The listing builds one solid part. Answer for the finished solid, in the listing's coordinates (mm). A direction names the side the tool comes from. Coordinates: 2 decimals unless noted, no trailing zeros. Order: outer loops, then holes, each group sorted by start corner. A loop starts at its lowest first (then second) coordinate and runs counter-clockwise, first axis right, second up. Notation, with made-up numbers: (69.5, 53.5) -> (104.5, 53.5) arc R19 cw to (104.5, 58.5) -> close; hole circle Ø2 at (6, -33). An arc over 180 degrees is marked (long way). Put each result on its own line as item: value. Start each with the question number.
```python
from build123d import *

# Parameters (mm, degrees)
EXTRUDE_1_DEPTH     = 1.63
SKETCH_2_R          = 1.5
CUT_EXTRUDE_1_DEPTH = 1.6
SKETCH_3_W          = 29.19
SKETCH_3_H          = 26.15
EXTRUDE_2_DEPTH     = 1.8
EXTRUDE_3_DEPTH     = 2
SKETCH_6_W          = 3
SKETCH_6_H          = 26.15
CUT_EXTRUDE_2_DEPTH = 0.2
SKETCH_4_W          = 5.81
SKETCH_4_H          = 3.67
EXTRUDE_4_DEPTH     = 2
SKETCH_7_W          = 2.6
SKETCH_7_H          = 1.3
EXTRUDE_5_DEPTH     = 1
SKETCH_8_W          = 51
SKETCH_8_H          = 5
EXTRUDE_6_DEPTH     = 3.68
SKETCH_9_W          = 1.9
SKETCH_9_H          = 1.9
EXTRUDE_7_DEPTH     = 3
SKETCH_10_R         = 1.6
EXTRUDE_8_DEPTH     = 1


with BuildPart() as part:
    # 草图1 → 凸台-拉伸1 (new body)
    with BuildSketch(Plane(origin=(0, 0, 0), x_dir=(1, 0, 0), z_dir=(0, 1, 0))):
        with BuildLine():
            Line((-29.5, 15.375), (29.5, 15.375))
            ThreePointArc((29.5, 15.375), (31.621320344, 14.496320344), (32.5, 12.375))
            Line((32.5, 12.375), (32.5, -12.375))
            ThreePointArc((32.5, -12.375), (31.621320344, -14.496320344), (29.5, -15.375))
            Line((29.5, -15.375), (-29.5, -15.375))
            ThreePointArc((-29.5, -15.375), (-31.621320344, -14.496320344), (-32.5, -12.375))
            Line((-32.5, -12.375), (-32.5, 12.375))
            ThreePointArc((-32.5, 12.375), (-31.621320344, 14.496320344), (-29.5, 15.375))
        make_face()
    extrude(amount=EXTRUDE_1_DEPTH)

    # 草图2 → 切除-拉伸1 (cut)
    with BuildSketch(Plane(origin=(0, 1.63, 0), x_dir=(1, 0, 0), z_dir=(0, 1, 0))):
        with Locations(Location((-29, 11.875, 0), (0, 0, 270))):
            Circle(SKETCH_2_R)
        with Locations(Location((-29, -11.875, 0), (0, 0, 270))):
            Circle(SKETCH_2_R)
        with Locations(Location((29, -11.875, 0), (0, 0, 270))):
            Circle(SKETCH_2_R)
        with Locations(Location((29, 11.875, 0), (0, 0, 270))):
            Circle(SKETCH_2_R)
    extrude(amount=-CUT_EXTRUDE_1_DEPTH, mode=Mode.SUBTRACT)

    # 草图3 → 凸台-拉伸2 (add)
    with BuildSketch(Plane(origin=(0, 1.63, 0), x_dir=(1, 0, 0), z_dir=(0, 1, 0))):
        with Locations((0.765, 1.1)):
            Rectangle(SKETCH_3_W, SKETCH_3_H)
    extrude(amount=EXTRUDE_2_DEPTH)

    # 草图5 → 凸台-拉伸3 (add)
    with BuildSketch(Plane(origin=(0, 1.63, 0), x_dir=(1, 0, 0), z_dir=(0, 1, 0))):
        with BuildLine():
            Line((26.574695167, 4.138250353), (29.014213562, 1.698731957))
            ThreePointArc((29.014213562, 1.698731957), (29.6, 0.284518395), (29.014213562, -1.129695167))
            Line((29.014213562, -1.129695167), (26.574695167, -3.569213562))
            ThreePointArc((26.574695167, -3.569213562), (25.160481605, -4.155), (23.746268043, -3.569213562))
            Line((23.746268043, -3.569213562), (21.306749647, -1.129695167))
            ThreePointArc((21.306749647, -1.129695167), (20.72096321, 0.284518395), (21.306749647, 1.698731957))
            Line((21.306749647, 1.698731957), (23.746268043, 4.138250353))
            ThreePointArc((23.746268043, 4.138250353), (25.160481605, 4.72403679), (26.574695167, 4.138250353))
        make_face()
    extrude(amount=EXTRUDE_3_DEPTH)

    # 草图6 → 切除-拉伸2 (cut)
    with BuildSketch(Plane(origin=(0, 3.43, 0), x_dir=(1, 0, 0), z_dir=(0, 1, 0))):
        with Locations((-12.33, 1.1)):
            Rectangle(SKETCH_6_W, SKETCH_6_H)
    extrude(amount=-CUT_EXTRUDE_2_DEPTH, mode=Mode.SUBTRACT)

    # 草图4 → 凸台-拉伸4 (add)
    with BuildSketch(Plane(origin=(0, 1.63, 0), x_dir=(1, 0, 0), z_dir=(0, 1, 0))):
        with Locations((-24.325, 6.14)):
            Rectangle(SKETCH_4_W, SKETCH_4_H)
        with Locations((-24.325, 0.27)):
            Rectangle(SKETCH_4_W, SKETCH_4_H)
        with Locations((-24.325, -5.6)):
            Rectangle(SKETCH_4_W, SKETCH_4_H)
    extrude(amount=EXTRUDE_4_DEPTH)

    # 草图7 → 凸台-拉伸5 (add)
    with BuildSketch(Plane(origin=(0, 3.63, 0), x_dir=(1, 0, 0), z_dir=(0, 1, 0))):
        with Locations((-24.325, 6.14)):
            Rectangle(SKETCH_7_W, SKETCH_7_H)
        with Locations((-24.325, 0.27)):
            Rectangle(SKETCH_7_W, SKETCH_7_H)
        with Locations((-24.325, -5.6)):
            Rectangle(SKETCH_7_W, SKETCH_7_H)
    extrude(amount=EXTRUDE_5_DEPTH)

    # 草图8 → 凸台-拉伸6 (add)
    with BuildSketch(Plane.XZ):
        with Locations((-0.2, -11.235)):
            Rectangle(SKETCH_8_W, SKETCH_8_H)
    extrude(amount=EXTRUDE_6_DEPTH)

    # 草图9 → 凸台-拉伸7 (add)
    with BuildSketch(Plane(origin=(0, 3.63, 0), x_dir=(1, 0, 0), z_dir=(0, 1, 0))):
        with Locations((25.160481605, 0.284518395)):
            Rectangle(SKETCH_9_W, SKETCH_9_H)
    extrude(amount=EXTRUDE_7_DEPTH)

    # 草图10 → 凸台-拉伸8 (add)
    with BuildSketch(Plane(origin=(0, 3.63, 0), x_dir=(1, 0, 0), z_dir=(0, 1, 0))):
        with Locations(Location((25.160481605, 0.284518395, 0), (0, 0, 90))):
            Circle(SKETCH_10_R)
    extrude(amount=EXTRUDE_8_DEPTH)


solid = part.part
```
(1) For a pull along X with two mould halves and no side action, classify faces 1 (the flat face through (-21.42, 3, 6)), 2 (the flat face through (-1, -2, -13.735)), 3 (the flat face through (24.21, 6, 0)) as released by +X, released by -X, zero draft, split by the parting line, or undercut.
(2) The part is cut by section A-A on x = -17.5. Determine the outline of the cut face in (y, z) (3 decimals).
(3) Find the intervals of material crossed by L1, parallel to Y at x = 23.5, z = 8.5; L2, parallel to X at y = 3.5, z = 0.5; L3, parallel to Y at x = 22.5, z = 1.5, in increasing order.
(4) The part is cut by section B-B on z = 11. Determine the outline of the cut face in (x, y).
(5) A tool of negligible diameter and unlimited length cuts with its end or side. For faces 4 (the flat face through (22.51, 2.62, -2.9)), 5 (the flat face through (1, 3, -14.175)), 6 (the flat face through (25.3, -2, -11)), 7 (the flat face through (-24, 3, -7.975)), from which of +Z, -Z, +X, -X, +Y, -Y can it reach the whole face along a straight path? Write none if from no direction.
(6) The part is cut by section D-D on x = 14. Determine the outline of the cut face in (y, z) (3 decimals), plus the area to 3 significant figures.
(7) Each of these flat-tipped pins is pushed along its axis until it touches: P1, Ø10, axis at x = -15.5, z = 0.5, coming from the +Y side; P2, Ø0.9, axis at x = 29, z = 12, coming from the +Y side; P3, Ø1, axis at x = -25, z = 0, coming from the +Y side; P4, Ø4, axis at x = 5, y = -0.5, coming from the +Z side (3 decimals). Where does it stop, or does it pass through?
(8) The part is cut by section C-C on y = -2. Determine the outline of the cut face in (x, z) (3 decimals), plus the area to 3 significant figures.
Worked out:
1. face 1: undercut
1. face 2: zero draft
1. face 3: released by -X
2. outline: (-3.68, -13.735) -> (0, -13.735) -> (0, -15.375) -> (1.63, -15.375) -> (1.63, 15.375) -> (0, 15.375) -> (0, -8.735) -> (-3.68, -8.735) -> close
3. L1: 0 to 1.63
3. L2: -27.23 to -21.42, 20.88 to 29.44
3. L3: 0 to 3.63
4. outline: (-32.5, 0) -> (32.5, 0) -> (32.5, 1.63) -> (30.22, 1.63) -> (30.22, 0.03) -> (27.78, 0.03) -> (27.78, 1.63) -> (15.36, 1.63) -> (15.36, 3.43) -> (-10.83, 3.43) -> (-10.83, 3.23) -> (-13.83, 3.23) -> (-13.83, 1.63) -> (-27.78, 1.63) -> (-27.78, 0.03) -> (-30.22, 0.03) -> (-30.22, 1.63) -> (-32.5, 1.63) -> close
5. face 4: -Z, +Y
5. face 5: -Z, +X, -X, +Y
5. face 6: +Z, -Z, +X, -Y
5. face 7: -Z, -X, +Y
6. outline: (-3.68, -13.735) -> (0, -13.735) -> (0, -15.375) -> (1.63, -15.375) -> (1.63, -14.175) -> (3.43, -14.175) -> (3.43, 11.975) -> (1.63, 11.975) -> (1.63, 15.375) -> (0, 15.375) -> (0, -8.735) -> (-3.68, -8.735) -> close
6. area: 116 mm2
7. P1: y = 3.43
7. P2: y = 0.03
7. P3: y = 4.63
7. P4: z = 15.375
8. outline: (-25.7, -13.735) -> (25.3, -13.735) -> (25.3, -8.735) -> (-25.7, -8.735) -> close
8. area: 255 mm2
